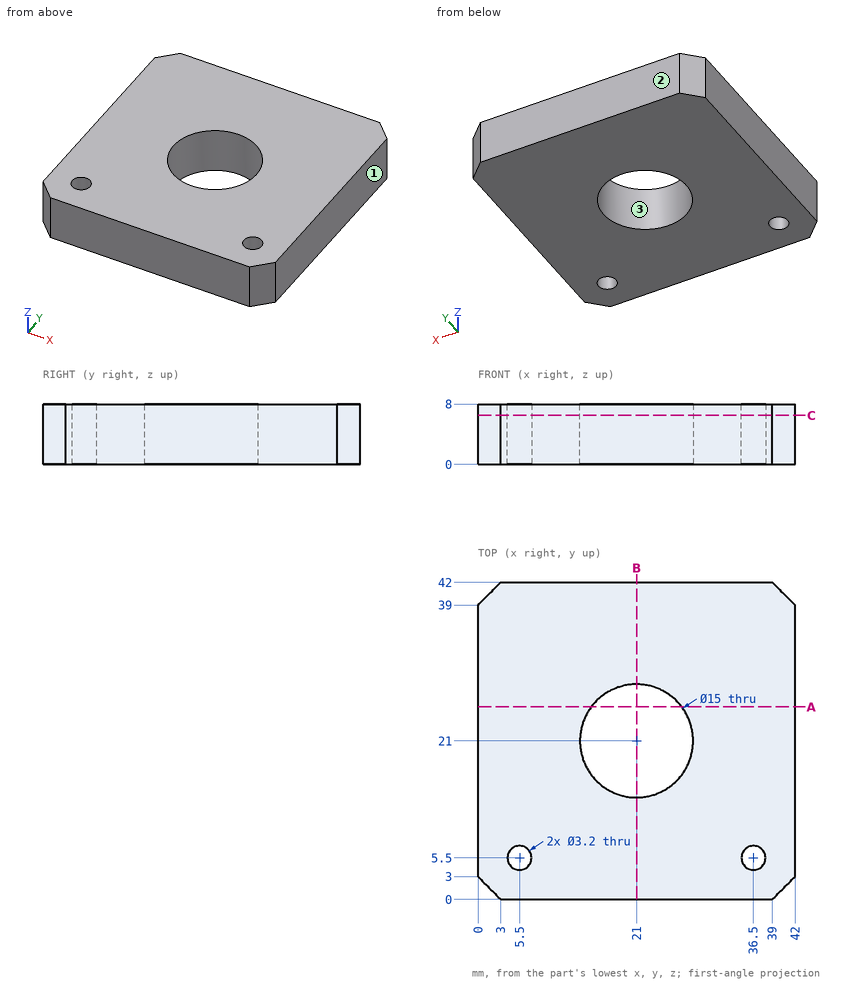
Print and shaded views of the part. All mm, measured from the part's lowest x, y and z. Round coordinates to 2 decimals unless told otherwise and drop trailing zeros. Loops run counter-clockwise (first coordinate to the right, second up) from the corner with the lowest first, then second, coordinate; pieces in that order, holes last. Notation, with made-up numbers: M -30,-15.75 L -3,-15.75 A18 cw -3,-1.75 Z; hole C 81.25,65 d10. An arc over 180 degrees is marked long. One line per question, with ' | ' between items.
1) Drill centre lines: line 1 along Y through (x, z) = (21, 7.5); line 2 along Y through (x, z) = (36.5, 5.25); line 3 along X through (y, z) = (22.5, 1.75). Where is each one in solid material? Low to high.
Solved:
line 1: y = 0 to 13.5, 28.5 to 42 | line 2: y = 0 to 3.9, 7.1 to 42 | line 3: x = 0 to 13.65, 28.35 to 42
2) Band-saw the part on C-C (z = 6.5). Give the cut face in (x, y).
Solved:
outline: M 0,3 L 3,0 L 39,0 L 42,3 L 42,39 L 39,42 L 3,42 L 0,39 Z; hole C 5.5,5.5 d3.2; hole C 21,21 d15; hole C 36.5,5.5 d3.2
3) Band-saw the part on B-B (x = 21). Give the cut face in (y, z).
Solved:
outline: M 0,0 L 13.5,0 L 13.5,8 L 0,8 Z; M 28.5,0 L 42,0 L 42,8 L 28.5,8 Z
4) Flat gauge pin, fed straight in: pin 1 (12 mm diameter, centred on x = 21, y = 21, fed in from -Z). Where does the tip first touch, or does it go through?
Solved:
pin 1: passes through
5) Band-saw the part on A-A (y = 25.5). Give the cut face in (x, z), then the cut area to 3 significant figures.
Solved:
outline: M 0,0 L 15,0 L 15,8 L 0,8 Z; M 27,0 L 42,0 L 42,8 L 27,8 Z | area: 240 mm²
6) Mould opens along Y. For the marked faces 1, 2 and 3 say: +Y half, -Y half, draft (parallel to the pull), parting line (faces both ways), or undercut.
Solved:
face 1: draft | face 2: +Y half | face 3: undercut
